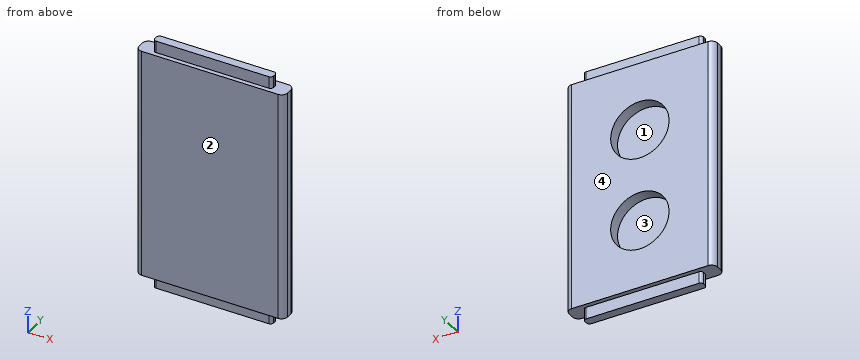
```python
from build123d import *

# Parameters (mm, degrees)
SKETCH1_W           = 63.5
SKETCH1_H           = 99.06
BOSS_EXTRUDE1_DEPTH = 7.62
SKETCH2_R           = 12.5
CUT_EXTRUDE1_DEPTH  = 5.08
FILLET1_R           = 2.54
SKETCH3_W           = 50.8
SKETCH3_H           = 3.81
BOSS_EXTRUDE2_DEPTH = 5.08
FILLET2_R           = 1.27
SKETCH4_W           = 50.8
SKETCH4_H           = 3.81
BOSS_EXTRUDE3_DEPTH = 5.08
FILLET3_R           = 1.27


with BuildPart() as part:
    # Sketch1 → Boss-Extrude1 (new body)
    with BuildSketch(Plane(origin=(0, 0, 0), x_dir=(1, 0, 0), z_dir=(0, 1, 0))):
        Rectangle(SKETCH1_W, SKETCH1_H)
    extrude(amount=BOSS_EXTRUDE1_DEPTH)

    # Sketch2 → Cut-Extrude1 (cut)
    with BuildSketch(Plane(origin=(0, 7.62, 0), x_dir=(1, 0, 0), z_dir=(0, 1, 0))):
        with Locations((0, -20.1)):
            Circle(SKETCH2_R)
        with Locations((0, 20.1)):
            Circle(SKETCH2_R)
    extrude(amount=-CUT_EXTRUDE1_DEPTH, mode=Mode.SUBTRACT)

    # Fillet1
    fillet1_edges = [part.edges().sort_by_distance(p)[0] for p in [
        (-31.75, 7.62, 0),
        (31.75, 7.62, 0),
        (-31.75, 0, 0),
        (31.75, 0, 0),
    ]]
    fillet(fillet1_edges, radius=FILLET1_R)

    # Sketch3 → Boss-Extrude2 (add)
    with BuildSketch(Plane.XY.offset(49.53)):
        with Locations((0, 3.81)):
            Rectangle(SKETCH3_W, SKETCH3_H)
    extrude(amount=BOSS_EXTRUDE2_DEPTH)

    # Fillet2
    fillet2_edges = [part.edges().sort_by_distance(p)[0] for p in [
        (-25.4, 5.715, 52.07),
        (-25.4, 1.905, 52.07),
        (25.4, 1.905, 52.07),
        (25.4, 5.715, 52.07),
    ]]
    fillet(fillet2_edges, radius=FILLET2_R)

    # Sketch4 → Boss-Extrude3 (add)
    with BuildSketch(Plane(origin=(0, 0, -49.53), x_dir=(-1, 0, 0), z_dir=(0, 0, -1))):
        with Locations((0, 3.772103496)):
            Rectangle(SKETCH4_W, SKETCH4_H)
    extrude(amount=BOSS_EXTRUDE3_DEPTH)

    # Fillet3
    fillet3_edges = [part.edges().sort_by_distance(p)[0] for p in [
        (-25.4, 1.867103496, -52.07),
        (-25.4, 5.677103496, -52.07),
        (25.4, 5.677103496, -52.07),
        (25.4, 1.867103496, -52.07),
    ]]
    fillet(fillet3_edges, radius=FILLET3_R)


solid = part.part
```
Could you check a few things on this model? Use its own coordinates, in mm. Face numbers are marked on the shaded views. A direction names the side the tool comes from. Coordinates: 2 decimals unless noted, no trailing zeros. Write each loop counter-clockwise with the first axis right and the second up, starting at its lowest first coordinate (ties: lowest second). Pieces come first, ordered by that corner, then holes. Notation, with made-up numbers: (39.25, 22) -> (81.25, 22) arc R38 ccw to (81.25, 61) -> close; hole circle Ø2 at (34.25, 55.5). An arc over 180 degrees is marked (long way). Write item = value, one per line. Start each with the question number.
(1) I want a section at B-B (z = 20.1). Please give me the cut outline in (x, y), plus the area to 3 significant figures.
(2) I want a section at A-A (x = -14.5). Please give me the cut outline in (y, z) (3 decimals).
(3) We'd pull the mould along Z, two halves only. Please class the marked faces 3 and 4: released by +Z, released by -Z, zero draft, split by the parting line, or undercut.
(4) Will these pins go through, and if not, where does the flat tip stop? pin 1 (2.5 mm diameter, centred on x = 6.5, z = 53.5, fed in from +Y) (3 decimals); pin 2 (0.6 mm diameter, centred on y = 3.5, z = -52, fed in from +X); pin 3 (7.5 mm diameter, centred on x = 2, z = 19, fed in from +Y).
(5) I want a section at C-C (x = 0). Please give me the cut outline in (y, z) (3 decimals), plus the area to 3 significant figures.
(6) I need wall thicknesses on line 1 (Z direction, x = 0, y = 6.4); line 2 (Z direction, x = 0, y = 4.1); line 3 (X direction, y = 4.55, z = -20.1). Which ranges of each line are inside material? Lowest first, please. Write a range as [from, to].
(7) Which directions (+Z, -Z, +X, -X, +Y, -Y) give clear straight access to the entire face, cutting with the end or side of a thin tool? Please do the marked faces 1 and 2.
Result set:
q1.outline = (-31.75, 2.54) arc R2.54 ccw to (-29.21, 0) -> (29.21, 0) arc R2.54 ccw to (31.75, 2.54) -> (31.75, 5.08) arc R2.54 ccw to (29.21, 7.62) -> (12.5, 7.62) -> (12.5, 2.54) -> (-12.5, 2.54) -> (-12.5, 7.62) -> (-29.21, 7.62) arc R2.54 ccw to (-31.75, 5.08) -> close
q1.area = 351 mm2
q2.outline = (0, -49.53) -> (1.867, -49.53) -> (1.867, -54.61) -> (5.677, -54.61) -> (5.677, -49.53) -> (7.62, -49.53) -> (7.62, 49.53) -> (5.715, 49.53) -> (5.715, 54.61) -> (1.905, 54.61) -> (1.905, 49.53) -> (0, 49.53) -> close
q3.face_3 = undercut
q3.face_4 = zero draft
q4.pin_1 = 5.715
q4.pin_2 = 25.4
q4.pin_3 = 2.54
q5.outline = (0, -49.53) -> (1.867, -49.53) -> (1.867, -54.61) -> (5.677, -54.61) -> (5.677, -49.53) -> (7.62, -49.53) -> (7.62, -32.6) -> (2.54, -32.6) -> (2.54, -7.6) -> (7.62, -7.6) -> (7.62, 7.6) -> (2.54, 7.6) -> (2.54, 32.6) -> (7.62, 32.6) -> (7.62, 49.53) -> (5.715, 49.53) -> (5.715, 54.61) -> (1.905, 54.61) -> (1.905, 49.53) -> (0, 49.53) -> close
q5.area = 540 mm2
q6.line_1 = [-49.53, -32.6], [-7.6, 7.6], [32.6, 49.53]
q6.line_2 = [-54.61, -32.6], [-7.6, 7.6], [32.6, 54.61]
q6.line_3 = [-31.75, -12.5], [12.5, 31.75]
q7.face_1 = +Y
q7.face_2 = +Z, -Z, +X, -X, -Y
